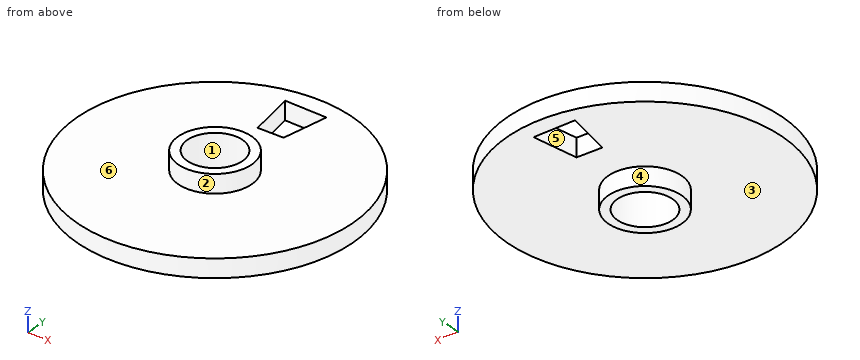
from build123d import *

# Parameters (mm, degrees)
SKETCH_1_R      = 4
SKETCH_1_R_2    = 3
EXTRUDE_1_DEPTH = 2
SKETCH_2_R      = 15
SKETCH_2_R_2    = 3
EXTRUDE_2_DEPTH = 2
SKETCH_3_R      = 4
SKETCH_3_R_2    = 3
EXTRUDE_3_DEPTH = 2


with BuildPart() as part:
    # Эскиз1 → Бобышка-Вытянуть1 (new body)
    with BuildSketch(Plane.XY):
        Circle(SKETCH_1_R)
        Circle(SKETCH_1_R_2, mode=Mode.SUBTRACT)
    extrude(amount=EXTRUDE_1_DEPTH)

    # Эскиз2 → Бобышка-Вытянуть2 (add)
    with BuildSketch(Plane.XY.offset(2)):
        Circle(SKETCH_2_R)
        Circle(SKETCH_2_R_2, mode=Mode.SUBTRACT)
        Polygon((-1.404174417, 7.963468844), (-2.307449736, 13.086197736), (2.292250749, 13), (1.410615846, 8), align=None, mode=Mode.SUBTRACT)
    extrude(amount=EXTRUDE_2_DEPTH)

    # Эскиз3 → Бобышка-Вытянуть3 (add)
    with BuildSketch(Plane.XY.offset(4)):
        Circle(SKETCH_3_R)
        Circle(SKETCH_3_R_2, mode=Mode.SUBTRACT)
    extrude(amount=EXTRUDE_3_DEPTH)


solid = part.part
Here's how the part is built. I have some questions about the finished solid (model axes, mm). Face numbers are marked on the shaded views. A direction names the side the tool comes from. Round coordinates to 2 decimals unless told otherwise and drop trailing zeros. Order: outer loops, then holes, each group sorted by start corner. A loop starts at its lowest first (then second) coordinate and runs counter-clockwise, first axis right, second up. Notation, with made-up numbers: (55, 51.25) -> (95, 51.25) arc R29 cw to (95, 87.25) -> close; hole circle Ø2 at (37.25, 68.25). An arc over 180 degrees is marked (long way). Return JSON: item names as keys, results as strings.
Q1. If we section it at D-D on z = 5.5: List the corners of the cut face in (x, y) for me.
Filled sheet:
{"outline": "circle Ø8 at (0, 0); hole circle Ø6 at (0, 0)"}
Q2. Which directions (+Z, -Z, +X, -X, +Y, -Y) give clear straight access to the entire face, cutting with the end or side of a thin tool? Please do the marked faces 4, 5 and 6.
Filled sheet:
{"face 4": "-Z", "face 5": "+Z, -Z", "face 6": "+Z"}
Q3. If we mould it in two halves opening along X, with no side actions, what happens to the marked faces 1, 2 and 3? For each: released by +X, released by -X, zero draft, split by the parting line, or undercut.
Filled sheet:
{"face 1": "undercut", "face 2": "split by the parting line", "face 3": "zero draft"}
Q4. If we section it at C-C on z = 3.15: List the corners of the cut face in (x, y) for me.
Filled sheet:
{"outline": "circle Ø30 at (0, 0); hole circle Ø6 at (0, 0); hole (-2.31, 13.09) -> (-1.4, 7.96) -> (1.41, 8) -> (2.29, 13) -> close"}
Q5. If we section it at B-B on x = 0: List the corners of the cut face in (y, z) for me, plus the area to 3 significant figures.
Filled sheet:
{"outline": "(-15, 2) -> (-4, 2) -> (-4, 0) -> (-3, 0) -> (-3, 6) -> (-4, 6) -> (-4, 4) -> (-15, 4) -> close; (3, 0) -> (4, 0) -> (4, 2) -> (7.98, 2) -> (7.98, 4) -> (4, 4) -> (4, 6) -> (3, 6) -> close; (13.04, 2) -> (15, 2) -> (15, 4) -> (13.04, 4) -> close", "area": "45.9 mm^2"}
Q6. For pin 1 Ø8 at (x, y) = (7.5, -7) entering from +Z; pin 2 Ø1.5 at (x, y) = (11, -12) entering from +Z; pin 3 Ø3 at (x, y) = (-2, -10) entering from -Z; pin 4 Ø3 at (y, z) = (11, 2) entering from +X, each with a flat end and sliding along its axis, tell me the tip position at first contact or that it passes through.
Filled sheet:
{"pin 1": "stops at z = 4", "pin 2": "passes through", "pin 3": "stops at z = 2", "pin 4": "stops at x = 11.61"}
Q7. I need wall thicknesses on line 1 along Y through (x, z) = (-0.75, 3.85); line 2 along Z through (x, y) = (-4, 5); line 3 along X through (y, z) = (2.5, 2.8). Which ranges of each line are inside material? Lowest first, please. Write a range as from..to.
Filled sheet:
{"line 1": "y = -14.98..-2.9, 2.9..7.97, 13.06..14.98", "line 2": "z = 2..4", "line 3": "x = -14.79..-1.66, 1.66..14.79"}
Q8. If we section it at A-A on y = 0: List the corners of the cut face in (x, z) for me.
Filled sheet:
{"outline": "(-15, 2) -> (-4, 2) -> (-4, 0) -> (-3, 0) -> (-3, 6) -> (-4, 6) -> (-4, 4) -> (-15, 4) -> close; (3, 0) -> (4, 0) -> (4, 2) -> (15, 2) -> (15, 4) -> (4, 4) -> (4, 6) -> (3, 6) -> close"}
